The model under review builds one solid part; all positions refer to its coordinate system, in mm. A direction names the side the tool comes from. Coordinates: 2 decimals unless noted, no trailing zeros. Loops run counter-clockwise (first coordinate to the right, second up) from the corner with the lowest first, then second, coordinate; pieces in that order, holes last. Notation, with made-up numbers: M 26.5,65.5 L 49.5,65.5 A26 cw 49.5,85.5 Z; hole C 73.25,8 d1. An arc over 180 degrees is marked long. Use one line per item in the form item = value.
```python
from build123d import *

# Parameters (mm, degrees)
F0_R     = 15
F1_DEPTH = 7
F2_DEPTH = 5
F3_SIZE  = 1


with BuildPart() as f1:
    # F0 (on Top) → F1 (new body)
    with BuildSketch(Plane.XY):
        Circle(F0_R)
        with BuildLine():
            ThreePointArc((1.254631, 1.22), (0, -1.75), (-1.254631, 1.22))
            Line((-1.254631, 1.22), (1.254631, 1.22))
        make_face(mode=Mode.SUBTRACT)
    extrude(amount=F1_DEPTH)

    # F0 (on Top) → F2 (join)
    with BuildSketch(Plane.XY):
        Circle(F0_R)
        with BuildLine():
            ThreePointArc((1.254631, 1.22), (0, -1.75), (-1.254631, 1.22))
            Line((-1.254631, 1.22), (1.254631, 1.22))
        make_face(mode=Mode.SUBTRACT)
    extrude(amount=F2_DEPTH)

    # F3
    f3_edges = [f1.edges().sort_by_distance(p)[0] for p in [
        (-15, 0, 0),
    ]]
    chamfer(f3_edges, length=F3_SIZE)


solid = f1.part
```
1. Add section B-B (y = 0). State the section outline as (x, z) points, then the cut area to 4 significant figures.
Response values:
outline = M -15,1 L -14,0 L -1.75,0 L -1.75,7 L -15,7 Z; M 1.75,0 L 14,0 L 15,1 L 15,7 L 1.75,7 Z
area = 184.5 mm^2
2. Add section A-A (x = 0). State the section outline as (y, z) points.
Response values:
outline = M -15,1 L -14,0 L -1.75,0 L -1.75,7 L -15,7 Z; M 1.22,0 L 14,0 L 15,1 L 15,7 L 1.22,7 Z
3. Wall thickness on line 1 along Y through (x, z) = (0, 2.25); line 2 along X through (y, z) = (-0.25, 2); line 3 along Y through (x, z) = (-7.25, 3): over which ranges is each line inside the solid? List them lowest first. Write a range as from..to.
Response values:
line_1 = -15..-1.75, 1.22..15
line_2 = -15..-1.73, 1.73..15
line_3 = -13.13..13.13
4. Insertion check: P1, Ø2, axis at x = 0, y = 0, coming from the -Z side; P2, Ø6, axis at x = 6, y = -7, coming from the -Z side; P3, Ø1, axis at x = 5.5, z = 3, coming from the +Y side; P4, Ø1, axis at y = 1.5, z = 3.5, coming from the -X side. Each pin has a flat end and moves straight along its axis. Give the tip position at first contact, or say it passes through.
Response values:
P1 = through
P2 = 0
P3 = 14.14
P4 = -14.97
5. Machinability: for faces 1 (the face through (3, 0, 7)), 2 (the face through (0, 1.22, 3)), which of the approach directions +Z, -Z, +X, -X, +Y, -Y give a long, thin tool a straight path to every point of the face, cutting with its end or side? Answer none if there is none.
Response values:
face_1 = +Z, +X, -X, +Y, -Y
face_2 = +Z, -Z
6. The part is to be moulded in two halves that separate along Y. For faces 3 (the face through (0, -3, 0)), 4 (the face through (-14.985, 0.66, 3.958)), 5 (the face through (0.06, -1.75, 3.45)), say which applies: pulls with the +Y half, pulls with the -Y half, needs draft (parallel to the pull), parting line crosses it, or undercut.
Response values:
face_3 = needs draft
face_4 = parting line crosses it
face_5 = undercut
